Source: CAD feature listing. Evaluate the final solid. Frame: model axes, mm. A direction names the side the tool comes from. Coordinates: 2 decimals unless noted, no trailing zeros. Order: outer loops, then holes, each group sorted by start corner. A loop starts at its lowest first (then second) coordinate and runs counter-clockwise, first axis right, second up. Notation, with made-up numbers: (55, 39) -> (75, 39) arc R26 cw to (75, 68) -> close; hole circle Ø11 at (-12.5, 17.25). An arc over 180 degrees is marked (long way). Put each result on its own line as item: value.
from build123d import *

# Parameters (mm, degrees)
F0_W     = 76.2
F0_H     = 38.1
F1_DEPTH = 25.4
F2_R     = 9.525
F3_DEPTH = 12.7
F4_SIZE2 = 3.175
F4_SIZE  = 3.175
F5_T     = 7.9375
F6_R     = 3.175
F7_DEPTH = 38.1


# Not quite as in the source:
# - a shell that OpenCascade refuses in one call is made with other operations: the cavity is built on its own and cut out


with BuildPart() as f1:
    # F0 (on Top) → F1 (new body)
    with BuildSketch(Plane.XY):
        with Locations((38.1, -19.05)):
            Rectangle(F0_W, F0_H)
    extrude(amount=F1_DEPTH)

    # F2 (on face) → F3 (join)
    with BuildSketch(Plane.XY.offset(25.4)):
        with Locations((57.15, -19.05)):
            Circle(F2_R)
        with Locations((19.05, -19.05)):
            Circle(F2_R)
    extrude(amount=F3_DEPTH)

    # F4
    f4_edges = [f1.edges().sort_by_distance(p)[0] for p in [
        (9.525, -19.05, 38.1),
        (47.625, -19.05, 38.1),
        (76.2, -19.05, 25.4),
        (38.1, -38.1, 25.4),
        (0, -19.05, 25.4),
        (38.1, 0, 25.4),
    ]]
    chamfer(f4_edges, length=F4_SIZE, length2=F4_SIZE2)

    # F5: shell of thickness 7.9375, made by hand


with BuildPart() as f5_core1:
    # F5_t2: copy of F1
    add(f1.part)

    # the walls: a layer under each face that stays
    f5_faces = [f5_core1.faces().sort_by_distance(p)[0] for p in [
        (38.1, 0, 11.1125),
        (76.2, -19.05, 11.1125),
        (38.1, -1.5875, 23.8125),
        (0, -19.05, 11.1125),
        (38.1, -38.1, 11.1125),
        (74.6125, -19.05, 23.8125),
        (38.1, -19.05, 25.4),
        (1.5875, -19.05, 23.8125),
        (38.1, -36.5125, 23.8125),
        (9.525, -19.05, 30.1625),
        (47.625, -19.05, 30.1625),
        (11.1125, -19.05, 36.5125),
        (49.2125, -19.05, 36.5125),
        (19.05, -19.05, 38.1),
        (57.15, -19.05, 38.1),
    ]]
    thicken(f5_faces, amount=-F5_T, mode=Mode.SUBTRACT)

    # F5_s3 → F5_t4 (revolve, cut)
    with BuildSketch(Plane.XZ.offset(19.05)):
        Polygon((28.654375, 25.479375), (28.575, 17.4625), (20.6375, 17.4625), (20.6375, 25.4), align=None)
    revolve(axis=Axis((19.05, -19.05, 25.4), (0, 0, 1)), mode=Mode.SUBTRACT)

    # F5_s5 → F5_t6 (revolve, cut)
    with BuildSketch(Plane.XZ.offset(19.05)):
        Polygon((66.754375, 25.479375), (66.675, 17.4625), (58.7375, 17.4625), (58.7375, 25.4), align=None)
    revolve(axis=Axis((57.15, -19.05, 25.4), (0, 0, 1)), mode=Mode.SUBTRACT)


with BuildPart() as f1_1:
    add(f1.part)

    # what is left inside the walls is the cavity
    f5_cavity = [f5_core1.part.solids().sort_by_distance(p)[0] for p in [
        (38.1, -22.754167, 0.079375),
    ]]
    add(f5_cavity, mode=Mode.SUBTRACT)

    # F6 (on face) → F7 (cut)
    with BuildSketch(Plane.XZ.offset(38.1)):
        with Locations((38.1, 12.7)):
            Circle(F6_R)
    extrude(amount=-F7_DEPTH, mode=Mode.SUBTRACT)


solid = f1_1.part
1. Set-up query: faces 4 (the flat face through (37.567, -36.49, 23.835)), 5 (the flat face through (38, -19, 25.4)), 6 (the flat face through (68.262, -19, 9)). Return all of +Z, -Z, +X, -X, +Y, -Y with unobstructed straight access to the full face (end or side cutting, diameter ignored); none if empty.
Numbers:
face 4: +Z, +X, -X, -Y
face 5: +Z
face 6: -Z
2. First-contact query: pin 1 (5 mm diameter, centred on x = 19.05, y = -19.05, fed in from -Z); pin 2 (10 mm diameter, centred on x = 33.5, y = -7, fed in from +Z); pin 3 (1 mm diameter, centred on x = 58, y = -19, fed in from -Z). Flat tips, straight axial feed; report the tip coordinate or a pass-through.
Numbers:
pin 1: stops at z = 17.46
pin 2: stops at z = 25.4
pin 3: stops at z = 30.16
3. Cut plane B-B on z = 12.7. Output: boundary loops of the cut face in (x, y) (1 decimal).
Numbers:
outline: (0, -38.1) -> (34.9, -38.1) -> (34.9, -30.2) -> (7.9, -30.2) -> (7.9, -7.9) -> (34.9, -7.9) -> (34.9, 0) -> (0, 0) -> close; (41.3, -38.1) -> (76.2, -38.1) -> (76.2, 0) -> (41.3, 0) -> (41.3, -7.9) -> (68.3, -7.9) -> (68.3, -30.2) -> (41.3, -30.2) -> close
4. Cut plane A-A on x = 38.1. Output: boundary loops of the cut face in (y, z) (1 decimal), plus the area to 3 significant figures.
Numbers:
outline: (-38.1, 0) -> (-30.2, 0) -> (-30.2, 9.5) -> (-38.1, 9.5) -> close; (-38.1, 15.9) -> (-30.2, 15.9) -> (-30.2, 17.5) -> (-7.9, 17.5) -> (-7.9, 15.9) -> (0, 15.9) -> (0, 22.2) -> (-3.2, 25.4) -> (-34.9, 25.4) -> (-38.1, 22.2) -> close; (-7.9, 0) -> (0, 0) -> (0, 9.5) -> (-7.9, 9.5) -> close
area: 469 mm2
5. Cut plane C-C on x = 19.05. Output: boundary loops of the cut face in (y, z) (1 decimal).
Numbers:
outline: (-38.1, 0) -> (-30.2, 0) -> (-30.2, 17.5) -> (-20.6, 17.5) -> (-20.6, 30.2) -> (-17.5, 30.2) -> (-17.5, 17.5) -> (-7.9, 17.5) -> (-7.9, 0) -> (0, 0) -> (0, 22.2) -> (-3.2, 25.4) -> (-9.5, 25.4) -> (-9.5, 34.9) -> (-12.7, 38.1) -> (-25.4, 38.1) -> (-28.6, 34.9) -> (-28.6, 25.4) -> (-34.9, 25.4) -> (-38.1, 22.2) -> close
6. Ray query, line 1 along X through (y, z) = (-30, 2); line 2 along X through (y, z) = (-19.05, 20.75); line 3 along Y through (x, z) = (9.5, 6). Return the intervals inside material, ascending.
Numbers:
line 1: x = 0 to 7.94, 68.26 to 76.2
line 2: x = 0 to 17.46, 20.64 to 55.56, 58.74 to 76.2
line 3: y = -38.1 to -30.16, -7.94 to 0
7. Pull-direction query (Y, two-part tool) for faces 1 (the conical face through (18.203, -12.601, 37.946)), 2 (the flat face through (57, -19, 38.1)), 3 (the flat face through (57, -19, 30.162)); classes: pulls with the +Y half, pulls with the -Y half, needs draft (parallel to the pull), parting line crosses it, or undercut.
Numbers:
face 1: parting line crosses it
face 2: needs draft
face 3: undercut
